Design review of the part built by this model. Coordinates are the model's own, in mm. A direction names the side the tool comes from. Give positions to 0.01 mm unless a question says otherwise; leave off trailing zeros. Order: outer loops, then holes, each group sorted by start corner. A loop starts at its lowest first (then second) coordinate and runs counter-clockwise, first axis right, second up. Notation, with made-up numbers: (24, -30) -> (37, -30) arc R26 ccw to (37, 3) -> close; hole circle Ø5 at (26.25, 87.5). An arc over 180 degrees is marked (long way). One line per item, written item: value. Start each with the question number.
1) Tool access review of faces 4 (the face through (0, 0, 0)), 5 (the face through (0.254, 13, -15)), 6 (the face through (6.56, 4.35, -8.09)), 7 (the face through (12.7, 0, 0)), 8 (the face through (6.724, 26.341, -17.364)): name each direction out of +Z, -Z, +X, -X, +Y, -Y from which nothing blocks a thin tool from reaching the whole face with its end or side.
2) For pin 1 (4.5 mm diameter, centred on y = 16.5, z = 8.5, fed in from -X); pin 2 (3 mm diameter, centred on x = 6.35, z = 0, fed in from +Y); pin 3 (2 mm diameter, centred on x = 6.35, z = -19.05, fed in from +Y), all flat-tipped, find the tip position at first contact; note any pin that passes through.
3) Consider section A-A (x = 3.25). State the section outline as (y, z) points, plus the area to 3 significant figures.
4) Consider section B-B (z = 6). State the section outline as (x, y) points, plus the area to 3 significant figures.
5) Consider section D-D (y = -12.7). State the section outline as (x, z) points, plus the area to 3 significant figures.
6) The part is to be moulded in two halves that separate along Y. For faces 1 (the face through (6.724, 26.341, 20.736)), 2 (the face through (6.56, 21.05, 8.09)), 3 (the face through (6, -31.75, 0)), say which applies: released by +Y, released by -Y, zero draft, split by the parting line, or undercut.
7) Wall thickness on line 1 along Z through (x, y) = (6.35, 23.75); line 2 along Y through (x, z) = (10.25, -12.5); line 3 along Y through (x, z) = (4.75, -9.5): over which ranges is each line inside the solid? List them lowest first. Write a range as from..to.
8) Consider section C-C (y = 6.5). State the section outline as (x, z) points.
from build123d import *

# Parameters (mm, degrees)
SKETCH1_W                  = 50.8
SKETCH1_H                  = 63.5
BOSS_EXTRUDE1_DEPTH        = 12.7
F_22_0_22_DIAMETER_HOLE1_D = 22
F_4_40_TAPPED_HOLE1_D      = 2.2606
CUT_EXTRUDE1_DEPTH         = 43.597094971
CUT_EXTRUDE2_DEPTH         = 0.254
F_8_32_TAPPED_HOLE1_D      = 3.4544
F_8_32_TAPPED_HOLE1_DEPTH  = 10.668
F_8_32_TAPPED_HOLE1_TIP    = 1.037806461


with BuildPart() as part:
    # Sketch1 → Boss-Extrude1 (new body)
    with BuildSketch(Plane(origin=(0, 0, 0), x_dir=(0, 0, -1), z_dir=(1, 0, 0))):
        Rectangle(SKETCH1_W, SKETCH1_H)
    extrude(amount=BOSS_EXTRUDE1_DEPTH)

    # Ø22.0 (22) Diameter Hole1 (through all)
    with Locations(Plane(origin=(12.7, 0, 0), x_dir=(0, 0, -1), z_dir=(1, 0, 0))):
        with Locations((0, -12.7)):
            Hole(F_22_0_22_DIAMETER_HOLE1_D / 2)

    # Sketch4 → 1/16 NPT Tapped Hole1 (revolve, cut)
    with BuildSketch(Plane.ZX.offset(12.7)):
        Polygon((0, 0), (0, 13.530685027), (3.0734, 11.684), (3.0734, 6.858), (3.762574096, 6.858), (3.9679118, 0), align=None)
    revolve(axis=Axis((-6.35, 12.7, 0), (1, 0, 0)), mode=Mode.SUBTRACT)

    # #4-40 Tapped Hole1 (through all)
    with Locations(Plane(origin=(12.7, 0, 0), x_dir=(0, 0, -1), z_dir=(1, 0, 0))):
        with Locations((-12.5, 12.7), (12.5, 12.7)):
            Hole(F_4_40_TAPPED_HOLE1_D / 2)

    # Sketch9 → Cut-Extrude1 (cut, through all)
    with BuildSketch(Plane(origin=(12.7, 0, 0), x_dir=(0, 0, -1), z_dir=(1, 0, 0))):
        with BuildLine():
            Line((-3.65, 2.54), (3.65, 2.54))
            ThreePointArc((3.65, 2.54), (8.140128061, 4.399871939), (10, 8.89))
            Line((10, 8.89), (10, 16.51))
            ThreePointArc((10, 16.51), (8.140128061, 21.000128061), (3.65, 22.86))
            Line((3.65, 22.86), (-3.65, 22.86))
            ThreePointArc((-3.65, 22.86), (-8.140128061, 21.000128061), (-10, 16.51))
            Line((-10, 16.51), (-10, 8.89))
            ThreePointArc((-10, 8.89), (-8.140128061, 4.399871939), (-3.65, 2.54))
        make_face()
    extrude(amount=-CUT_EXTRUDE1_DEPTH, mode=Mode.SUBTRACT)

    # Sketch10 → Cut-Extrude2 (cut)
    with BuildSketch(Plane(origin=(0, 0, 0), x_dir=(0, 0, -1), z_dir=(1, 0, 0))):
        with BuildLine():
            Line((-12.5, 2.54), (12.5, 2.54))
            ThreePointArc((12.5, 2.54), (16.990128061, 4.399871939), (18.85, 8.89))
            Line((18.85, 8.89), (18.85, 16.51))
            ThreePointArc((18.85, 16.51), (16.990128061, 21.000128061), (12.5, 22.86))
            Line((12.5, 22.86), (-12.5, 22.86))
            ThreePointArc((-12.5, 22.86), (-16.990128061, 21.000128061), (-18.85, 16.51))
            Line((-18.85, 16.51), (-18.85, 8.89))
            ThreePointArc((-18.85, 8.89), (-16.990128061, 4.399871939), (-12.5, 2.54))
        make_face()
    extrude(amount=CUT_EXTRUDE2_DEPTH, mode=Mode.SUBTRACT)

    # #8-32 Tapped Hole1
    with Locations(Plane(origin=(0, 31.75, 0), x_dir=(1, 0, 0), z_dir=(0, 1, 0))):
        with Locations((6.35, 19.05), (6.35, -19.05), (6.35, 0)):
            Hole(F_8_32_TAPPED_HOLE1_D / 2, depth=F_8_32_TAPPED_HOLE1_DEPTH)
            with Locations((0, 0, -(F_8_32_TAPPED_HOLE1_DEPTH + F_8_32_TAPPED_HOLE1_TIP / 2))):  # 118° drill point
                Cone(0, F_8_32_TAPPED_HOLE1_D / 2, F_8_32_TAPPED_HOLE1_TIP, mode=Mode.SUBTRACT)


solid = part.part
Checked values:
1. face 4: +Z, -Z, -X, +Y, -Y
1. face 5: -X
1. face 6: +X, -X
1. face 7: +Z, -Z, +X, +Y, -Y
1. face 8: +Y
2. pin 1: stops at x = 0.25
2. pin 2: stops at y = 2.54
2. pin 3: stops at y = 20.65
3. outline: (-31.75, -25.4) -> (31.75, -25.4) -> (31.75, 25.4) -> (-31.75, 25.4) -> close; hole circle Ø22 at (-12.7, 0); hole (2.54, -3.65) arc R6.35 ccw to (8.89, -10) -> (16.51, -10) arc R6.35 ccw to (22.86, -3.65) -> (22.86, 3.65) arc R6.35 ccw to (16.51, 10) -> (8.89, 10) arc R6.35 ccw to (2.54, 3.65) -> close; hole circle Ø2.26 at (12.7, -12.5); hole circle Ø2.26 at (12.7, 12.5)
3. area: 2,470 mm^2
4. outline: (0, -31.75) -> (12.7, -31.75) -> (12.7, -21.92) -> (0, -21.92) -> close; (0, -3.48) -> (12.7, -3.48) -> (12.7, 2.99) -> (0.25, 2.99) -> (0.25, 2.54) -> (0, 2.54) -> close; (0, 22.86) -> (0.25, 22.86) -> (0.25, 22.41) -> (12.7, 22.41) -> (12.7, 31.75) -> (0, 31.75) -> close
4. area: 325 mm^2
5. outline: (0, -25.4) -> (12.7, -25.4) -> (12.7, -11) -> (0, -11) -> close; (0, 11) -> (12.7, 11) -> (12.7, 25.4) -> (0, 25.4) -> close
5. area: 366 mm^2
6. face 1: zero draft
6. face 2: undercut
6. face 3: released by -Y
7. line 1: z = -25.4..-20.78, -17.32..-1.73, 1.73..17.32, 20.78..25.4
7. line 2: y = -31.75..11.57, 13.83..31.75
7. line 3: y = -31.75..-18.25, -7.15..6.42, 18.98..31.75
8. outline: (0, -25.4) -> (12.7, -25.4) -> (12.7, -9.53) -> (0.25, -9.53) -> (0.25, -18.38) -> (0, -18.38) -> close; (0, 18.38) -> (0.25, 18.38) -> (0.25, 9.53) -> (12.7, 9.53) -> (12.7, 25.4) -> (0, 25.4) -> close
